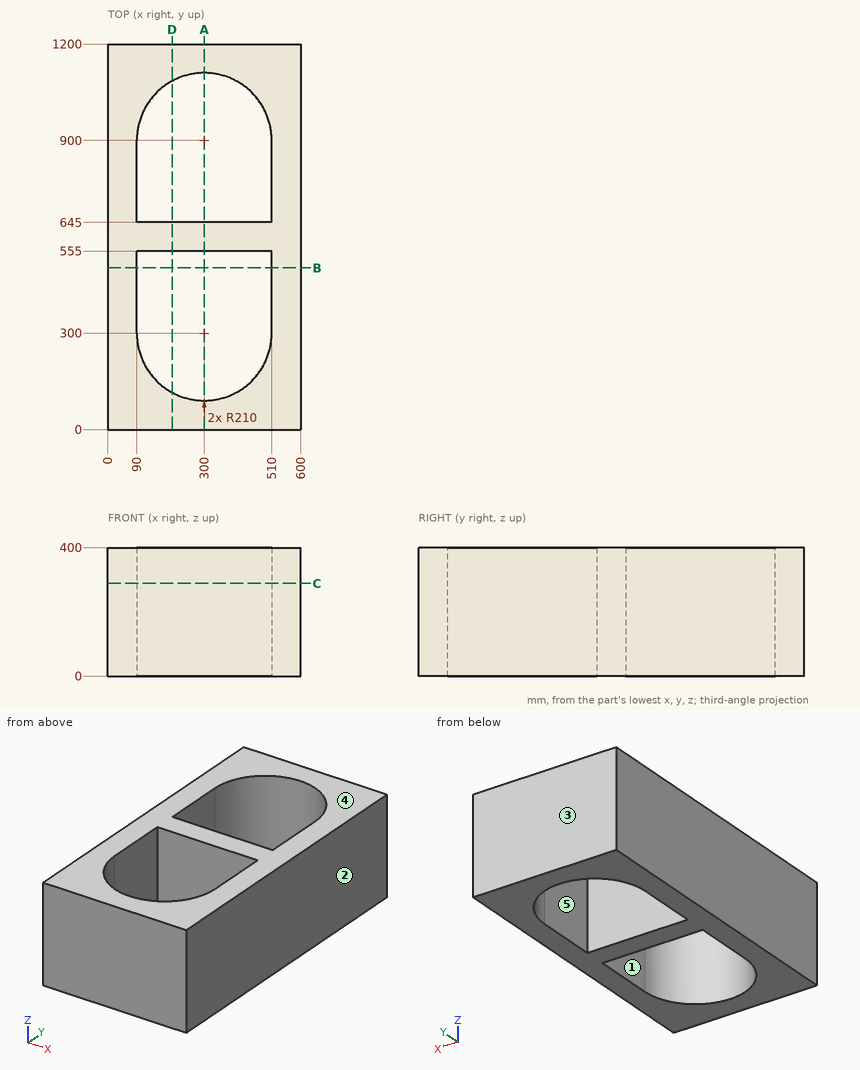
Answer from the drawing. Dimensions are ordinates in mm from the lowest x, y and z of the part. A direction names the side the tool comes from. Coordinates: 2 decimals unless noted, no trailing zeros. Loops run counter-clockwise (first coordinate to the right, second up) from the corner with the lowest first, then second, coordinate; pieces in that order, holes last.
1) For a pull along Y with two mould halves and no side action, classify the marked faces 3, 4 and 5 as +Y half, -Y half, draft (parallel to the pull), parting line (faces both ways), or undercut.
Results:
face 3: +Y half
face 4: draft
face 5: undercut
2) Section D-D (x = 200) is taken. Give the vertices of the cut face in (y, z), plus the area to 3 significant figures.
Results:
outline: (0, 0) - (115.34, 0) - (115.34, 400) - (0, 400) - close; (555, 0) - (645, 0) - (645, 400) - (555, 400) - close; (1084.66, 0) - (1200, 0) - (1200, 400) - (1084.66, 400) - close
area: 128,000 mm2
3) Section C-C (z = 288.5) is taken. Give the vertices of the cut face in (x, y), plus the area to 3 significant figures.
Results:
outline: (0, 0) - (600, 0) - (600, 1200) - (0, 1200) - close; hole (90, 300) arc R210 ccw to (510, 300) - (510, 555) - (90, 555) - close; hole (90, 645) - (510, 645) - (510, 900) arc R210 ccw to (90, 900) - close
area: 367,000 mm2
4) Consider probe 1 along X at (y, z) = (665.5, 164.5); probe 2 along Y at (x, z) = (395.5, 273.5); probe 3 along Y at (x, z) = (321, 348.5). Determine where each line is inside the solid, lowest interval first.
Results:
probe 1: x = 0 to 90, 510 to 600
probe 2: y = 0 to 112.97, 555 to 645, 1087.03 to 1200
probe 3: y = 0 to 91.05, 555 to 645, 1108.95 to 1200
5) Section A-A (x = 300) is taken. Give the vertices of the cut face in (y, z), plus the area to 3 significant figures.
Results:
outline: (0, 0) - (90, 0) - (90, 400) - (0, 400) - close; (555, 0) - (645, 0) - (645, 400) - (555, 400) - close; (1110, 0) - (1200, 0) - (1200, 400) - (1110, 400) - close
area: 108,000 mm2
6) A flat-ended cylindrical pin translates along its axis: pin 1 (12 mm diameter, centred on y = 529.5, z = 137.5, fed in from -X). Find the tip coordinate at first contact, or state that the pin passes through.
Results:
pin 1: stops at x = 0
7) Section B-B (y = 503) is taken. Give the vertices of the cut face in (x, z), plus the area to 3 significant figures.
Results:
outline: (0, 0) - (90, 0) - (90, 400) - (0, 400) - close; (510, 0) - (600, 0) - (600, 400) - (510, 400) - close
area: 72,000 mm2
8) For the marked faces 1 and 2, determine the directions among +Z, -Z, +X, -X, +Y, -Y from which every point of the face is accessible in a straight line to the end or side of a thin tool.
Results:
face 1: +Z, -Z
face 2: +Z, -Z, +X, +Y, -Y
